Geometry check sheet. Reference: the model listing, model coordinates, mm. A direction names the side the tool comes from. Coordinates: 2 decimals unless noted, no trailing zeros. Loops run counter-clockwise (first coordinate to the right, second up) from the corner with the lowest first, then second, coordinate; pieces in that order, holes last. Notation, with made-up numbers: M 56,-10 L 79,-10 A17 cw 79,6 Z; hole C 15.5,-29 d10. An arc over 180 degrees is marked long. Use CSV: the item, a comma, the result in double quotes.
```python
from build123d import *

# Parameters (mm, degrees)
SKETCH_1_W                  = 66
SKETCH_1_H                  = 56
EXTRUDE_1_DEPTH             = 10
SKETCH_2_W                  = 61
SKETCH_2_H                  = 51
CUT_EXTRUDE_1_DEPTH         = 7
SKETCH_3_R                  = 1.6
CUT_EXTRUDE_2_DEPTH         = 44.840620434
PATTERN_LINEAR_1_COUNT      = 2
PATTERN_LINEAR_1_PITCH      = 50
PATTERN_LINEAR_1_COUNT_DIR2 = 2
PATTERN_LINEAR_1_PITCH_DIR2 = 40
SKETCH_4_W                  = 40
SKETCH_4_H                  = 10.5
SKETCH_4_W_2                = 10.5
SKETCH_4_H_2                = 30
CUT_EXTRUDE_3_DEPTH         = 44.840620434
SKETCH_6_W                  = 14
SKETCH_6_H                  = 7
CUT_EXTRUDE_6_DEPTH         = 10
SKETCH_7_W                  = 14
SKETCH_7_H                  = 3
CUT_EXTRUDE_7_DEPTH         = 10


with BuildPart() as part:
    # 草图1 → 凸台-拉伸1 (new body)
    with BuildSketch(Plane(origin=(0, 0, 0), x_dir=(1, 0, 0), z_dir=(0, 1, 0))):
        Rectangle(SKETCH_1_W, SKETCH_1_H)
    extrude(amount=EXTRUDE_1_DEPTH)

    # 草图2 → 切除-拉伸1 (cut)
    with BuildSketch(Plane(origin=(0, 10, 0), x_dir=(1, 0, 0), z_dir=(0, 1, 0))):
        Rectangle(SKETCH_2_W, SKETCH_2_H)
    extrude(amount=-CUT_EXTRUDE_1_DEPTH, mode=Mode.SUBTRACT)

    # 草图3 → 切除-拉伸2 (cut, through all)
    with BuildSketch(Plane(origin=(0, 3, 0), x_dir=(1, 0, 0), z_dir=(0, 1, 0))):
        with Locations(Location((-25, 20, 0), (0, 0, 270))):
            Circle(SKETCH_3_R)
    cut_extrude_2 = extrude(amount=-CUT_EXTRUDE_2_DEPTH, mode=Mode.SUBTRACT)

    # 阵列(线性)1: Cut-Extrude 2 2 × 2
    with Locations(*[(i * PATTERN_LINEAR_1_PITCH, 0, j * PATTERN_LINEAR_1_PITCH_DIR2) for i in range(PATTERN_LINEAR_1_COUNT) for j in range(PATTERN_LINEAR_1_COUNT_DIR2) if (i, j) != (0, 0)]):
        add(cut_extrude_2, mode=Mode.SUBTRACT)

    # 草图4 → 切除-拉伸3 (cut, through all)
    with BuildSketch(Plane(origin=(0, 3, 0), x_dir=(1, 0, 0), z_dir=(0, 1, 0))):
        with Locations((0, 20.25)):
            Rectangle(SKETCH_4_W, SKETCH_4_H)
        with Locations((-25.25, 0)):
            Rectangle(SKETCH_4_W_2, SKETCH_4_H_2)
        Rectangle(SKETCH_4_W, SKETCH_4_H_2)
        with Locations((0, -20.25)):
            Rectangle(SKETCH_4_W, SKETCH_4_H)
        with Locations((25.25, 0)):
            Rectangle(SKETCH_4_W_2, SKETCH_4_H_2)
    extrude(amount=-CUT_EXTRUDE_3_DEPTH, mode=Mode.SUBTRACT)

    # 草图6 → 切除-拉伸6 (cut)
    with BuildSketch(Plane(origin=(-30.5, 0, 0), x_dir=(0, 0, -1), z_dir=(1, 0, 0))):
        with Locations((7.5, 6.5)):
            Rectangle(SKETCH_6_W, SKETCH_6_H)
    extrude(amount=-CUT_EXTRUDE_6_DEPTH, mode=Mode.SUBTRACT)

    # 草图7 → 切除-拉伸7 (cut)
    with BuildSketch(Plane(origin=(33, 0, 0), x_dir=(0, 0, -1), z_dir=(1, 0, 0))):
        with Locations((0, 8.5)):
            Rectangle(SKETCH_7_W, SKETCH_7_H)
    extrude(amount=-CUT_EXTRUDE_7_DEPTH, mode=Mode.SUBTRACT)


solid = part.part
```
1. Thickness scan on line 1 (X direction, y = 1.4, z = 20); line 2 (Z direction, x = -18.5, y = 5.5); line 3 (X direction, y = 9.75, z = -19). Record the ranges inside material, lowest first. Write a range as [from, to].
The answers:
line 1,"[-33, -26.6], [-23.4, -20], [20, 23.4], [26.6, 33]"
line 2,"[-28, -25.5], [25.5, 28]"
line 3,"[-33, -30.5], [30.5, 33]"
2. Gauge pin test, flat ends, axial feed: P1, Ø2.5, axis at x = -25, z = -20, coming from the +Y side; P2, Ø4, axis at x = 25, z = 20, coming from the +Y side; P3, Ø0.8, axis at x = 31.5, z = 0.5, coming from the +Y side. Record the tip position at first contact, or that the pin passes through.
The answers:
P1,"through"
P2,"y = 3"
P3,"y = 7"
3. Section check D-D, the plane x = 25. Record the cut outline in (y, z), plus the area to 3 significant figures.
The answers:
outline,"M 0,-28 L 10,-28 L 10,-25.5 L 3,-25.5 L 3,-21.6 L 0,-21.6 Z; M 0,-18.4 L 3,-18.4 L 3,-15 L 0,-15 Z; M 0,15 L 3,15 L 3,18.4 L 0,18.4 Z; M 0,21.6 L 3,21.6 L 3,25.5 L 10,25.5 L 10,28 L 0,28 Z"
area,"93.8 mm^2"
4. Set-up check for faces 5 (the flat face through (0, 5, 25.5)), 6 (the flat face through (0, 0, 27)), 7 (the flat face through (-33, 5, 0)), 8 (the flat face through (32, 7, 0)), 9 (the flat face through (20, 2, 20)): record each of +Z, -Z, +X, -X, +Y, -Y from which the full face is reachable in a straight line by a thin tool's end or side.
The answers:
face 5,"+Y"
face 6,"+Z, -Z, +X, -X, -Y"
face 7,"+Z, -Z, -X, +Y, -Y"
face 8,"+X, +Y"
face 9,"+Y, -Y"
5. Section check B-B, the plane x = 6.5. Record the cut outline in (y, z), plus the area to 3 significant figures.
The answers:
outline,"M 0,-28 L 10,-28 L 10,-25.5 L 0,-25.5 Z; M 0,25.5 L 10,25.5 L 10,28 L 0,28 Z"
area,"50.0 mm^2"
6. Release check for a two-part mould opening along Z. For faces 1 (the flat face through (25, 2, 15)), 2 (the flat face through (0, 5, 28)), 3 (the flat face through (0, 5, -28)), 4 (the flat face through (-3, 10, 26)) record: +Z half, -Z half, draft (parallel to the pull), parting line (faces both ways), or undercut.
The answers:
face 1,"undercut"
face 2,"+Z half"
face 3,"-Z half"
face 4,"draft"
7. Section check A-A, the plane z = 20. Record the cut outline in (x, y).
The answers:
outline,"M -33,0 L -26.6,0 L -26.6,3 L -30.5,3 L -30.5,10 L -33,10 Z; M -23.4,0 L -20,0 L -20,3 L -23.4,3 Z; M 20,0 L 23.4,0 L 23.4,3 L 20,3 Z; M 26.6,0 L 33,0 L 33,10 L 30.5,10 L 30.5,3 L 26.6,3 Z"
8. Section check C-C, the plane z = -10.5. Record the cut outline in (x, y).
The answers:
outline,"M -33,0 L -30.5,0 L -30.5,3 L -33,3 Z; M 30.5,0 L 33,0 L 33,10 L 30.5,10 Z"
